Read the model definition and answer for the solid it produces. Units are mm, in the model's axes. Face numbers are marked on the shaded views. A direction names the side the tool comes from. Give positions to 0.01 mm unless a question says otherwise; leave off trailing zeros. Loops run counter-clockwise (first coordinate to the right, second up) from the corner with the lowest first, then second, coordinate; pieces in that order, holes last. Notation, with made-up numbers: (7, 75.5) - (30, 75.5) arc R21 ccw to (30, 90.5) - close; hole circle Ø4 at (8, 6). An arc over 180 degrees is marked (long way). Write item = value, one per line. Start each with the question number.
Autodesk Inventor part; units mm, degrees
ref_plane "YZ Plane" through (0, 0, 0) normal (1, 0, 0) x (0, 1, 0)
ref_plane "XZ Plane" through (0, 0, 0) normal (0, 1, 0) x (-1, 0, 0)
ref_plane "XY Plane" through (0, 0, 0) normal (0, 0, 1) x (1, 0, 0)
sketch "Sketch1" plane through (0, 0, 0) normal (0, 0, 1) x (1, 0, 0)
  line L0 (0, 0) -> (10.2, 0)
  line L1 (10.2, 0) -> (10.2, 6)
  line L2 (10.2, 6) -> (0, 6)
  line L3 (0, 6) -> (0, 0)
  circle A0 centre (8.4, 4.5) radius 0.9
  line L4 (10.2, 3.5) -> (10.9353, 3.5)
  line L5 (10.9353, 3.5) -> (10.9353, 2.5)
  line L6 (10.9353, 2.5) -> (10.2, 2.5)
  line L7 (10.2, 2.5) -> (10.2, 3.5)
  line L8 (10.2, 3.5) -> (10.15, 3.5866)
  line L9 (10.15, 3.5866) -> (13.35, 5.4341)
  line L10 (13.35, 5.4341) -> (13.4, 5.3475)
  line L11 (13.4, 5.3475) -> (10.2, 3.5)
  line L12 (10.2, 2.5) -> (10.15, 2.4134)
  line L13 (10.15, 2.4134) -> (13.35, 0.5659)
  line L14 (13.35, 0.5659) -> (13.4, 0.6525)
  line L15 (13.4, 0.6525) -> (10.2, 2.5)
  circle A1 centre (1.9, 1.7) radius 0.75
  line L16 (0, 4.3634) -> (-2.5124, 6.3094)
  line L17 (-2.5124, 6.3094) -> (-1.2876, 7.8906)
  line L18 (-1.2876, 7.8906) -> (1.1531, 6)
  arc A2 (-1.2876, 7.8906) -> (-2.5124, 6.3094) centre (-1.9, 7.1) ccw
  point P0 (10.9353, 3)
  point P1 (10.2, 3)
  dimension "d0" = 10.2
  dimension "d1" = 6
  dimension "d2" = 1.8
  dimension "d3" = 1.5
  dimension "d4" = 1.8
  dimension "d5" = 2.8
  dimension "d6" = 6.5
  dimension "d7" = 1.5
  dimension "d8" = 0.1
  dimension "d9" = 0.1
  dimension "d10" = 2.1
  dimension "d11" = 13.1
  dimension "d12" = 30
  dimension "d13" = 30
  dimension "d15" = 1
  dimension "d16" = 5
  dimension "d17" = 2
extrude "Extrusion1" add sketch "Sketch1" along normal mid plane 4.2 contours L3 L2 L1 L9 L8 L12 L13 L0 | L13 L12 L1 | L8 L9 L1
extrude "Extrusion2" add sketch "Sketch1" along normal mid plane 1.8 contours L13 L12 L1 | L1 L15 L14 L13 | L1 L4 L5 L6 | L8 L9 L1 | L1 L9 L10 L11
extrude "Extrusion3" add sketch "Sketch1" along normal mid plane 5.8 contours A1
extrude "Extrusion4" add sketch "Sketch1" along normal mid plane 2 contours L16 L17 L18 L2 L3 | A2 L17
sketch "Sketch2" plane through (10.2, 2.5, 0.9) normal (0.5, 0.866, 0) x (0.866, -0.5, 0)
  line L0 (0, 0) -> (0, 1.8)
  line L1 (3.695, 0) -> (0, 0)
  line L2 (3.695, 1.8) -> (3.695, 0)
  line L3 (0, 1.8) -> (3.695, 1.8)
  line L4 (2.795, 0.9) -> (3.695, 0.9) construction
  point P0 (-7.5835, 0.9)
  dimension "d26" = 0.9
  dimension "d27" = 0.9
sketch "Sketch3" plane through (13.4, 5.3475, -0.9) normal (0.5, -0.866, 0) x (0.866, 0.5, 0)
  line L0 (0, 0) -> (0, 1.8)
  line L1 (-3.695, 1.8) -> (0, 1.8)
  line L2 (-3.695, 0) -> (-3.695, 1.8)
  line L3 (0, 0) -> (-3.695, 0)
  line L4 (0, 0) -> (0, 1.8) construction
  line L5 (0, 0.9) -> (-0.9, 0.9) construction
  point P0 (-14.2785, 0.9)
  dimension "d28" = 0.9
  dimension "d29" = 0.9
equation "\"d27\" = d26"
equation "\"d29\" = d28"
properties part number "LimitSwitch" material "ABS Plastic"
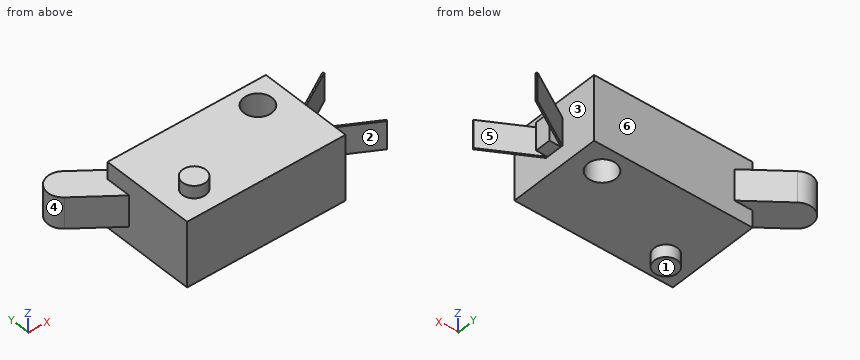
1. Consider line 1 along Y through (x, z) = (8.4, -1); line 2 along X through (y, z) = (1.75, -1.3); line 3 along Y through (x, z) = (3.75, 1.65). Determine where each line is inside the solid, lowest interval first. Write a range as [from, to].
2. A cutting plane is placed at A-A on x = 8.4. Give the vertices of the cut face in (y, z), and give its area (3 significant figures).
3. A cutting plane is placed at D-D on x = 1.9. Give the vertices of the cut face in (y, z).
4. Given P1, Ø2, axis at y = 4, z = 1, coming from the +X side; P2, Ø0.8, axis at x = 10.5, z = 0.5, coming from the +Y side; P3, Ø1.5, axis at x = 12, y = 4, coming from the -Z side, each flat-ended and moving along its own axis, determine where each tip first touches the part or whether it passes through.
5. A tool of negligible diameter and unlimited length cuts with its end or side. For the marked faces 1 and 2, from which of +Z, -Z, +X, -X, +Y, -Y can it reach the whole face along a straight path? Write none if from no direction.
6. A cutting plane is placed at C-C on y = 2.75. Give the vertices of the cut face in (x, z), and give its area (3 significant figures).
7. For a pull along X with two mould halves and no side action, classify the marked faces 3, 4, 5 and 6 as released by +X, released by -X, zero draft, split by the parting line, or undercut.
8. A cutting plane is placed at B-B on z = 0.4. Give the vertices of the cut face in (x, y), and give its area (3 significant figures).
Reply:
q1.line_1 = [0, 3.6], [5.4, 6]
q1.line_2 = [0, 10.2]
q1.line_3 = [0, 6]
q2.outline = (0, -2.1) - (3.6, -2.1) - (3.6, 2.1) - (0, 2.1) - close; (5.4, -2.1) - (6, -2.1) - (6, 2.1) - (5.4, 2.1) - close
q2.area = 17.6 mm^2
q3.outline = (0, -2.1) - (0.95, -2.1) - (0.95, -2.9) - (2.45, -2.9) - (2.45, -2.1) - (6, -2.1) - (6, 2.1) - (2.45, 2.1) - (2.45, 2.9) - (0.95, 2.9) - (0.95, 2.1) - (0, 2.1) - close
q4.P1 = 12.79
q4.P2 = 6
q4.P3 = -0.9
q5.face_1 = -Z, +X, -X, +Y, -Y
q5.face_2 = +Z, -Z, -Y
q6.outline = (0, -2.1) - (10.2, -2.1) - (10.2, -0.9) - (10.94, -0.9) - (10.94, 0.9) - (10.2, 0.9) - (10.2, 2.1) - (0, 2.1) - close
q6.area = 44.2 mm^2
q7.face_3 = undercut
q7.face_4 = split by the parting line
q7.face_5 = released by +X
q7.face_6 = zero draft
q8.outline = (-2.51, 6.31) - (0, 4.36) - (0, 0) - (10.2, 0) - (10.2, 2.38) - (13.35, 0.57) - (13.4, 0.65) - (10.2, 2.5) - (10.94, 2.5) - (10.94, 3.5) - (10.2, 3.5) - (13.4, 5.35) - (13.35, 5.43) - (10.2, 3.62) - (10.2, 6) - (1.15, 6) - (-1.29, 7.89) arc R1 ccw to start; hole circle Ø1.8 at (8.4, 4.5)
q8.area = 67.0 mm^2
